from build123d import *

# Parameters (mm, degrees)
EXTRUDE_1_DEPTH     = 1.35
SKETCH_8_W          = 18.4
SKETCH_8_H          = 16.75
EXTRUDE_4_DEPTH     = 4.75
SKETCH_2_R          = 1.575
EXTRUDE_2_DEPTH     = 1.6
SKETCH_4_W          = 18.6
SKETCH_4_H          = 14.85
EXTRUDE_3_DEPTH     = 3.3
SKETCH_3_W          = 14.7
SKETCH_3_H          = 12.15
CUT_EXTRUDE_1_DEPTH = 10.4
SKETCH_5_W          = 0.675
SKETCH_5_H          = 12.15
CUT_EXTRUDE_2_DEPTH = 0.8
SKETCH_6_R          = 0.75
CUT_EXTRUDE_3_DEPTH = 8.7


with BuildPart() as part:
    # Эскиз1 → Бобышка-Вытянуть1 (new body)
    with BuildSketch(Plane.XY):
        with BuildLine():
            Line((-12.75, -8.375), (12.75, -8.375))
            ThreePointArc((12.75, -8.375), (14.164213562, -7.789213562), (14.75, -6.375))
            Line((14.75, -6.375), (14.75, 6.375))
            ThreePointArc((14.75, 6.375), (14.164213562, 7.789213562), (12.75, 8.375))
            Line((12.75, 8.375), (-12.75, 8.375))
            ThreePointArc((-12.75, 8.375), (-14.164213562, 7.789213562), (-14.75, 6.375))
            Line((-14.75, 6.375), (-14.75, -6.375))
            ThreePointArc((-14.75, -6.375), (-14.164213562, -7.789213562), (-12.75, -8.375))
        make_face()
    extrude(amount=EXTRUDE_1_DEPTH)

    # Эскиз8 → Бобышка-Вытянуть4 (add)
    with BuildSketch(Plane(origin=(0, 0, 0), x_dir=(-1, 0, 0), z_dir=(0, 0, -1))):
        Rectangle(SKETCH_8_W, SKETCH_8_H)
    extrude(amount=EXTRUDE_4_DEPTH)

    # Эскиз2 → Бобышка-Вытянуть2 (add)
    with BuildSketch(Plane.XY.offset(1.35)):
        with Locations((-11.65, 3.5)):
            Circle(SKETCH_2_R)
        with Locations((11.65, 3.5)):
            Circle(SKETCH_2_R)
        with Locations((11.65, -3.5)):
            Circle(SKETCH_2_R)
        with Locations((-11.65, -3.5)):
            Circle(SKETCH_2_R)
    extrude(amount=EXTRUDE_2_DEPTH)

    # Эскиз4 → Бобышка-Вытянуть3 (add)
    with BuildSketch(Plane.XY.offset(1.35)):
        Rectangle(SKETCH_4_W, SKETCH_4_H)
    extrude(amount=EXTRUDE_3_DEPTH)

    # Эскиз3 → Вырез-Вытянуть1 (cut, through all)
    with BuildSketch(Plane.XY.offset(4.65)):
        Rectangle(SKETCH_3_W, SKETCH_3_H)
    extrude(amount=-CUT_EXTRUDE_1_DEPTH, mode=Mode.SUBTRACT)

    # Эскиз5 → Вырез-Вытянуть2 (cut)
    with BuildSketch(Plane.XY.offset(4.65)):
        with BuildLine():
            Line((-5.25, 6.65), (5.25, 6.65))
            ThreePointArc((5.25, 6.65), (5.825, 6.075), (5.25, 5.5))
            Line((5.25, 5.5), (-5.25, 5.5))
            ThreePointArc((-5.25, 5.5), (-5.825, 6.075), (-5.25, 6.65))
        make_face()
        with BuildLine():
            Line((-5.25, -6.65), (5.25, -6.65))
            ThreePointArc((5.25, -6.65), (5.825, -6.075), (5.25, -5.5))
            Line((5.25, -5.5), (-5.25, -5.5))
            ThreePointArc((-5.25, -5.5), (-5.825, -6.075), (-5.25, -6.65))
        make_face()
        with Locations((-7.6875, 0)):
            Rectangle(SKETCH_5_W, SKETCH_5_H)
        with Locations((7.6875, 0)):
            Rectangle(SKETCH_5_W, SKETCH_5_H)
    extrude(amount=-CUT_EXTRUDE_2_DEPTH, mode=Mode.SUBTRACT)

    # Эскиз6 → Вырез-Вытянуть3 (cut, through all)
    with BuildSketch(Plane.XY.offset(2.95)):
        with Locations((-11.65, 3.5)):
            Circle(SKETCH_6_R)
        with Locations((-11.65, -3.5)):
            Circle(SKETCH_6_R)
        with Locations((11.65, 3.5)):
            Circle(SKETCH_6_R)
        with Locations((11.65, -3.5)):
            Circle(SKETCH_6_R)
    extrude(amount=-CUT_EXTRUDE_3_DEPTH, mode=Mode.SUBTRACT)


solid = part.part
CAD build for the part. Positions are in the model's coordinates, mm. A direction names the side the tool comes from. Coordinates: 2 decimals unless noted, no trailing zeros. Order: outer loops, then holes, each group sorted by start corner. A loop starts at its lowest first (then second) coordinate and runs counter-clockwise, first axis right, second up.
Item 1: Two-plate mould, pull along X, no slides. Class faces 1 (the face through (0, 7.425, 3)), 2 (the face through (-12.811, -2.436, 2.139)), 3 (the face through (-14.75, 0, 1)): +X half, -X half, draft (parallel to the pull), parting line (faces both ways), or undercut.
Check sheet entries:
face 1: draft
face 2: undercut
face 3: -X half
Item 2: Band-saw the part on B-B on x = -1.25. List the corners of the cut face in (y, z) (3 decimals).
Check sheet entries:
outline: (-8.375, -4.75) - (-6.075, -4.75) - (-6.075, 3.85) - (-6.65, 3.85) - (-6.65, 4.65) - (-7.425, 4.65) - (-7.425, 1.35) - (-8.375, 1.35) - close; (6.075, -4.75) - (8.375, -4.75) - (8.375, 1.35) - (7.425, 1.35) - (7.425, 4.65) - (6.65, 4.65) - (6.65, 3.85) - (6.075, 3.85) - close
Item 3: Band-saw the part on D-D on x = -11.65. List the corners of the cut face in (y, z) (3 decimals), plus the area to 3 significant figures.
Check sheet entries:
outline: (-8.375, 0) - (-4.25, 0) - (-4.25, 2.95) - (-5.075, 2.95) - (-5.075, 1.35) - (-8.375, 1.35) - close; (-2.75, 0) - (2.75, 0) - (2.75, 2.95) - (1.925, 2.95) - (1.925, 1.35) - (-1.925, 1.35) - (-1.925, 2.95) - (-2.75, 2.95) - close; (4.25, 0) - (8.375, 0) - (8.375, 1.35) - (5.075, 1.35) - (5.075, 2.95) - (4.25, 2.95) - close
area: 23.8 mm2
Item 4: Band-saw the part on A-A on z = 2.5. Give the number of separate pieces and of enclosed holes in the cut face, plus the area to 3 significant figures.
Check sheet entries:
separate pieces: 5
enclosed holes: 5
area: 122 mm2
Item 5: Drill centre lines: L1, parallel to Y at x = -11.65, z = 1.1 (3 decimals); L2, parallel to X at y = 2, z = 3.25; L3, parallel to Y at x = -7, z = 0 (3 decimals). Where is each one in solid material? Low to high.
Check sheet entries:
L1: y = -8.375 to -4.25, -2.75 to 2.75, 4.25 to 8.375
L2: x = -9.3 to -7.35, 7.35 to 9.3
L3: y = -8.375 to -6.075, 6.075 to 8.375
Item 6: 3-axis set-ups, long thin cutter, end or side, ignore diameter. For faces 4 (the face through (14.18, 7.774, 0.666)), 5 (the face through (-12.4, 3.5, 1.5)), 6 (the face through (-9.3, 0, 3)), 7 (the face through (9.2, 0, -2)), 8 (the face through (12.497, 4.828, 2.139)): which of +Z, -Z, +X, -X, +Y, -Y reach the whole face in a straight line?
Check sheet entries:
face 4: +Z, -Z, +X, +Y
face 5: +Z, -Z
face 6: +Z, +Y, -Y
face 7: -Z, +X, +Y, -Y
face 8: +Z
Item 7: Pin check, flat tips, straight feed: pin 1 Ø4 at (y, z) = (6, -2.5) entering from -X; pin 2 Ø2 at (x, z) = (-9, 2.5) entering from +Y (3 decimals); pin 3 Ø1.6 at (y, z) = (-2.5, 2.5) entering from +X; pin 4 Ø1.2 at (x, y) = (11.65, 3.5) entering from +Z. Stop position of each tip, or through.
Check sheet entries:
pin 1: stops at x = -9.2
pin 2: stops at y = 7.425
pin 3: stops at x = 13.21
pin 4: passes through
Item 8: Band-saw the part on C-C on y = 1. List the corners of the cut face in (x, z) (3 decimals).
Check sheet entries:
outline: (-14.75, 0) - (-9.2, 0) - (-9.2, -4.75) - (-7.35, -4.75) - (-7.35, 3.85) - (-8.025, 3.85) - (-8.025, 4.65) - (-9.3, 4.65) - (-9.3, 1.35) - (-14.75, 1.35) - close; (7.35, -4.75) - (9.2, -4.75) - (9.2, 0) - (14.75, 0) - (14.75, 1.35) - (9.3, 1.35) - (9.3, 4.65) - (8.025, 4.65) - (8.025, 3.85) - (7.35, 3.85) - close
